```python
from build123d import *

# Parameters (mm, degrees)
SKETCH1_R           = 2.1
SKETCH1_R_2         = 1.6
BOSS_EXTRUDE1_DEPTH = 6.35
SKETCH2_W           = 18
SKETCH2_H           = 11
BOSS_EXTRUDE2_DEPTH = 14
SKETCH3_R           = 5.5
CUT_EXTRUDE1_DEPTH  = 3
CHAMFER1_SIZE       = 3
FILLET2_R           = 10
FILLET3_R           = 5
CUT_EXTRUDE2_DEPTH  = 2
SKETCH5_R           = 1.6
CUT_EXTRUDE3_DEPTH  = 2638.157111638
SKETCH6_R           = 2.95
CUT_EXTRUDE4_DEPTH  = 3


with BuildPart() as part:
    # Sketch1 → Boss-Extrude1 (new body)
    with BuildSketch(Plane(origin=(251.886129178, -2636.030473787, -0.277944786), x_dir=(1, 0, 0), z_dir=(0, 1, 0))):
        Polygon((-265.886129178, -0.277944786), (-251.886129178, -0.277944786), (-251.886129178, 59.722055214), (-306.886129178, 59.722055214), (-306.886129178, 40.722055214), align=None)
        with Locations(Location((-261.886129178, 8.722055214, 0), (0, 0, 270))):
            Circle(SKETCH1_R, mode=Mode.SUBTRACT)
        with Locations(Location((-282.886129178, 29.222055214, 0), (0, 0, 270))):
            Circle(SKETCH1_R_2, mode=Mode.SUBTRACT)
        with Locations(Location((-262.886129178, 49.722055214, 0), (0, 0, 270))):
            Circle(SKETCH1_R_2, mode=Mode.SUBTRACT)
        with Locations(Location((-277.886129178, 49.722055214, 0), (0, 0, 270))):
            Circle(SKETCH1_R_2, mode=Mode.SUBTRACT)
    extrude(amount=BOSS_EXTRUDE1_DEPTH)

    # Sketch2 → Boss-Extrude2 (add)
    with BuildSketch(Plane(origin=(-55, -2629.680473787, -60), x_dir=(1, 0, 0), z_dir=(0, -1, 0))):
        with Locations((9, 5.5)):
            Rectangle(SKETCH2_W, SKETCH2_H)
    extrude(amount=-BOSS_EXTRUDE2_DEPTH)

    # Sketch3 → Cut-Extrude1 (cut)
    with BuildSketch(Plane.XY.offset(-49)):
        with Locations((-47, -2623.180473787)):
            Circle(SKETCH3_R)
    extrude(amount=-CUT_EXTRUDE1_DEPTH, mode=Mode.SUBTRACT)

    # Chamfer1
    # the kernel refuses this chamfer: 3 mm, written as the material it adds along each edge
    with BuildSketch(Plane(origin=(-37, -2629.680473787, -49), x_dir=(0, -0.02749587661065579, 0.9996219169112949), z_dir=(-1, 0, 0))) as chamfer1_piece_1_section:
        Polygon((CHAMFER1_SIZE * 0.999621916911, CHAMFER1_SIZE * 0.0274958766107), (-CHAMFER1_SIZE * 0.0274958766107, CHAMFER1_SIZE * 0.999621916911), (0, 0), align=None)
    chamfer1_piece_1 = extrude(amount=18, mode=Mode.PRIVATE)
    chamfer1_piece_1 = chamfer1_piece_1 - Plane(origin=(-47, -2623.180473787, -47.945016367), x_dir=(1, 0, 0), z_dir=(0, 0, 1)) * Cylinder(5.5, 48, mode=Mode.PRIVATE)
    add(chamfer1_piece_1)
    with BuildSketch(Plane(origin=(-37, -2629.680473787, -60), x_dir=(0.9996219169112948, -0.027495876610655785, 0), z_dir=(0, 0, 1))) as chamfer1_piece_2:
        Polygon((CHAMFER1_SIZE * 0.999621916911, CHAMFER1_SIZE * 0.0274958766107), (-CHAMFER1_SIZE * 0.0274958766107, CHAMFER1_SIZE * 0.999621916911), (0, 0), align=None)
    extrude(amount=11)
    with BuildSketch(Plane(origin=(-29.284951036, -2629.680473787, -49), x_dir=(0, -0.02749587661065579, 0.9996219169112949), z_dir=(-1, 0, 0))) as chamfer1_piece_3a_section:
        Polygon((CHAMFER1_SIZE * 0.999621916911, CHAMFER1_SIZE * 0.0274958766107), (-CHAMFER1_SIZE * 0.0274958766107, CHAMFER1_SIZE * 0.999621916911), (0, 0), align=None)
    chamfer1_piece_3a = extrude(amount=25.715048964, mode=Mode.PRIVATE)
    chamfer1_piece_3a = split(chamfer1_piece_3a, bisect_by=Plane(origin=(-37, -2628.691092907, -48.01061912), z_dir=(1, 0, 0)), keep=Keep.TOP, mode=Mode.PRIVATE)
    with BuildSketch(Plane(origin=(-37, -2629.680473787, -60), x_dir=(0.9996219169112948, -0.027495876610655785, 0), z_dir=(0, 0, 1))) as chamfer1_piece_3b_section:
        Polygon((CHAMFER1_SIZE * 0.999621916911, CHAMFER1_SIZE * 0.0274958766107), (-CHAMFER1_SIZE * 0.0274958766107, CHAMFER1_SIZE * 0.999621916911), (0, 0), align=None)
    chamfer1_piece_3b = extrude(amount=18.715048964, mode=Mode.PRIVATE)
    chamfer1_piece_3b = split(chamfer1_piece_3b, bisect_by=Plane(origin=(-36.01061912, -2628.691092907, -49), z_dir=(0, 0, 1)), keep=Keep.TOP, mode=Mode.PRIVATE)
    chamfer1_piece_3 = chamfer1_piece_3a & chamfer1_piece_3b
    add(chamfer1_piece_3)

    # Fillet2
    # the kernel refuses this fillet: 10 mm, written as the material it takes off along each edge
    with BuildSketch(Plane(origin=(-14, -2646.385812847, 0), x_dir=(1, 0, 0), z_dir=(0, 1, 0)), Plane(origin=(-55, -2646.385812847, -41), x_dir=(0.7071067811865518, 0, 0.7071067811865432), z_dir=(0, 1, 0))) as fillet2_piece_1:
        with BuildLine():
            CenterArc((FILLET2_R * 0.414213562373, FILLET2_R), FILLET2_R, 225, 45)
            Line((-FILLET2_R * 0.292893218813, FILLET2_R * 0.292893218813), (0, 0))
            Line((0, 0), (FILLET2_R * 0.414213562373, 0))
        make_face()
    extrude(amount=27.060678119, mode=Mode.SUBTRACT)
    with BuildSketch(Plane(origin=(0, -2661.030473787, 0), x_dir=(0, 0, -1), z_dir=(0, 1, 0))) as fillet2_piece_2:
        with BuildLine():
            CenterArc((FILLET2_R, FILLET2_R), FILLET2_R, 180, 90)
            Line((0, FILLET2_R), (0, 0))
            Line((0, 0), (FILLET2_R, 0))
        make_face()
    extrude(amount=56.35, mode=Mode.SUBTRACT)

    # Fillet3
    fillet3_edges = [part.edges().sort_by_distance(p)[0] for p in [
        (-37, -2615.680473787, -54.5),
        (-55, -2615.680473787, -54.5),
    ]]
    fillet(fillet3_edges, radius=FILLET3_R)

    # Sketch4 → Cut-Extrude2 (cut)
    with BuildSketch(Plane.XY.offset(-52)):
        Polygon((-45.383419246, -2625.980473787), (-43.766838493, -2623.180473787), (-45.383419246, -2620.380473787), (-48.616580754, -2620.380473787), (-50.233161507, -2623.180473787), (-48.616580754, -2625.980473787), align=None)
    extrude(amount=-CUT_EXTRUDE2_DEPTH, mode=Mode.SUBTRACT)

    # Sketch5 → Cut-Extrude3 (cut, through all)
    with BuildSketch(Plane.XY.offset(-54)):
        with Locations((-47, -2623.180473787)):
            Circle(SKETCH5_R)
    extrude(amount=-CUT_EXTRUDE3_DEPTH, mode=Mode.SUBTRACT)

    # Sketch6 → Cut-Extrude4 (cut)
    with BuildSketch(Plane(origin=(0, 0, -60), x_dir=(-1, 0, 0), z_dir=(0, 0, -1))):
        with Locations((47, -2623.180473787)):
            Circle(SKETCH6_R)
    extrude(amount=-CUT_EXTRUDE4_DEPTH, mode=Mode.SUBTRACT)


solid = part.part
```
The model under review builds one solid part; all positions refer to its coordinate system, in mm. A direction names the side the tool comes from. Round coordinates to 2 decimals unless told otherwise and drop trailing zeros. Loops run counter-clockwise (first coordinate to the right, second up) from the corner with the lowest first, then second, coordinate; pieces in that order, holes last. Notation, with made-up numbers: (84, 61) -> (136, 61) arc R8 cw to (136, 73) -> close; hole circle Ø11 at (87, -26.75). An arc over 180 degrees is marked (long way). Answer as a JSON object with one key per item and string values. Group by question number.
1) Mouldability with a two-part tool opening along Y and no side actions: class faces 4 (the face through (-49.414, -2621.761, -52.986)), 5 (the face through (-37, -2624, -55)), 6 (the face through (-35.48, -2628.2, -53.1)) as released by +Y, released by -Y, zero draft, split by the parting line, or undercut.
2) We need section B-B on x = -31. Write out the cut boundary in (y, z).
3) For line 1 (X direction, y = -2634.75, z = -50); line 2 (Y direction, x = -47, z = -50.6); line 3 (Y direction, x = -3.5, z = -8), list the stretches that pass through material, from the lowest coordinate up. Write a range as [from, to].
4) We need section D-D on x = -11. Write out the cut boundary in (y, z), then the cut area to 3 significant figures.
5) For pin 1 Ø10 at (x, y) = (-47, -2623.18) entering from -Z; pin 2 Ø5 at (x, y) = (-21, -2629.5) entering from +Z; pin 3 Ø10 at (y, z) = (-2621, -6) entering from -X (3 decimals); pin 4 Ø4.5 at (x, y) = (-47.5, -2624) entering from +Z, all flat-tipped, find the tip position at first contact; note any pin that passes through.
6) We need section C-C on z = -29.5. Write out the cut boundary in (x, y), then the cut area to 3 significant figures.
7) We need section A-A on z = -50. Write out the cut boundary in (x, y), then the cut area to 3 significant figures.
8) For faces 1 (the face through (-48.3, -2624.5, -57)), 2 (the face through (-35, -2633, -21)), 3 (the face through (-47, -2620.38, -53)), list the 3-axis set-ups (+Z, -Z, +X, -X, +Y, -Y) from which the entire face can be reached by the end or side of a thin tool; tool diameter is ignored.
Result set:
{
 "1": {"face 4": "undercut", "face 5": "zero draft", "face 6": "released by +Y"},
 "2": {"outline": "(-2636.03, -60) -> (-2629.68, -60) -> (-2629.68, -31.1) -> (-2636.03, -31.1) -> close; (-2636.03, -27.9) -> (-2629.68, -27.9) -> (-2629.68, -17) -> (-2636.03, -17) -> close"},
 "3": {"line 1": "[-55, -27.6], [-24.4, -12.6], [-9.4, 0]", "line 2": "[-2636.03, -2628.68], [-2617.68, -2615.68]", "line 3": "[-2636.03, -2629.68]"},
 "4": {"outline": "(-2636.03, -60) -> (-2629.68, -60) -> (-2629.68, -51.6) -> (-2636.03, -51.6) -> close; (-2636.03, -48.4) -> (-2629.68, -48.4) -> (-2629.68, -10.85) -> (-2636.03, -10.85) -> close; (-2636.03, -7.15) -> (-2629.68, -7.15) -> (-2629.68, -0.07) -> (-2636.03, -0.07) -> close", "area": "337 mm²"},
 "5": {"pin 1": "z = -60", "pin 2": "z = -4.51", "pin 3": "through", "pin 4": "z = -52"},
 "6": {"outline": "(-43.5, -2636.03) -> (-32.6, -2636.03) -> (-32.6, -2629.68) -> (-43.5, -2629.68) -> close; (-29.4, -2636.03) -> (0, -2636.03) -> (0, -2629.68) -> (-29.4, -2629.68) -> close", "area": "256 mm²"},
 "7": {"outline": "(-55, -2636.03) -> (-27.6, -2636.03) -> (-27.6, -2629.68) -> (-34, -2629.68) -> (-37, -2626.68) -> (-37, -2620.68) arc R5 ccw to (-42, -2615.68) -> (-50, -2615.68) arc R5 ccw to (-55, -2620.68) -> close; (-24.4, -2636.03) -> (-12.6, -2636.03) -> (-12.6, -2629.68) -> (-24.4, -2629.68) -> close; (-9.4, -2636.03) -> (0, -2636.03) -> (0, -2629.68) -> (-9.4, -2629.68) -> close; hole circle Ø11 at (-47, -2623.18)", "area": "459 mm²"},
 "8": {"face 1": "-Z", "face 2": "+Z, -X, +Y, -Y", "face 3": "+Z"}
}
